Design review of the part shown in the three views and the two pictorial views. Dimensions are in mm from the part's minimum x, y and z. Round coordinates to 2 decimals unless told otherwise and drop trailing zeros. Order: outer loops, then holes, each group sorted by start corner. A loop starts at its lowest first (then second) coordinate and runs counter-clockwise, first axis right, second up.
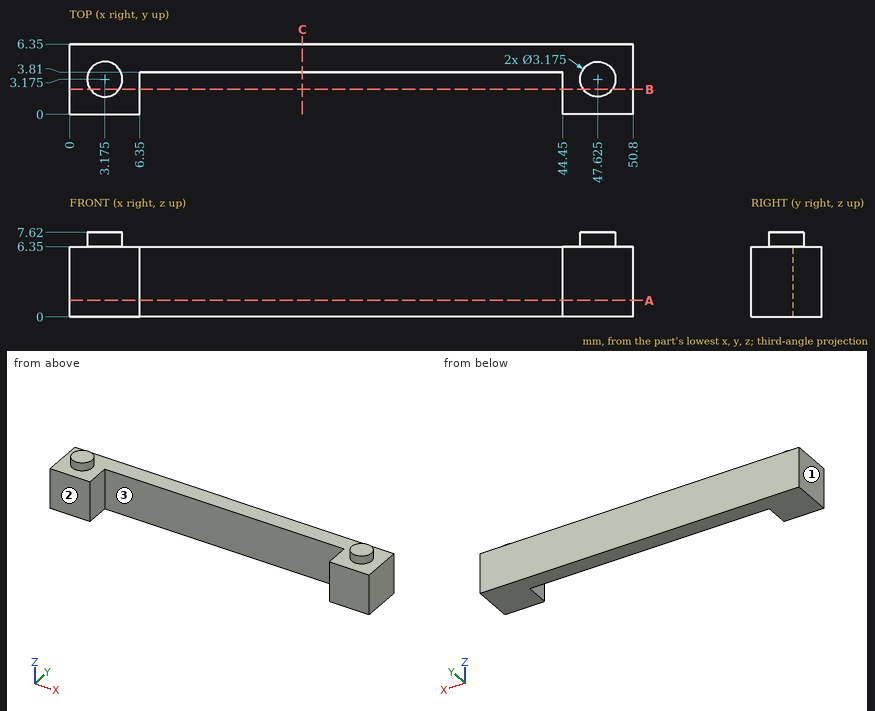
(1) Draft analysis for pull direction X (two halves, no side actions). For the marked faces 1, 2 and 3, state which applies: pulls with the +X half, pulls with the -X half, needs draft (parallel to the pull), parting line crosses it, or undercut.
(2) Clearance check with flat-ended pins moving along their axes: P1, Ø3, axis at x = 29, z = 1, coming from the -Y side; P2, Ø3, axis at x = 27, y = 5.5, coming from the +Z side. State where each tip first meets the part, or that it passes through.
(3) Add section A-A on z = 1.5. Give the boundary of the cut face in (x, y).
(4) Wall thickness on L1, parallel to X at y = 0.75, z = 3.5; L2, parallel to Z at x = 38, y = 5.5; L3, parallel to Y at x = 28.5, z = 5.75: over which ranges is each line inside the solid? List them lowest first.
(5) Add section C-C on x = 21. Give the boundary of the cut face in (y, z).
(6) Add section B-B on y = 2.25. Give the boundary of the cut face in (x, z).
Here are the results:
1. face 1: pulls with the -X half
1. face 2: needs draft
1. face 3: undercut
2. P1: stops at y = 3.81
2. P2: stops at z = 6.35
3. outline: (0, 0) - (6.35, 0) - (6.35, 3.81) - (44.45, 3.81) - (44.45, 0) - (50.8, 0) - (50.8, 6.35) - (0, 6.35) - close
4. L1: x = 0 to 6.35, 44.45 to 50.8
4. L2: z = 0 to 6.35
4. L3: y = 3.81 to 6.35
5. outline: (3.81, 0) - (6.35, 0) - (6.35, 6.35) - (3.81, 6.35) - close
6. outline: (0, 0) - (6.35, 0) - (6.35, 6.35) - (4.47, 6.35) - (4.47, 7.62) - (1.88, 7.62) - (1.88, 6.35) - (0, 6.35) - close; (44.45, 0) - (50.8, 0) - (50.8, 6.35) - (48.92, 6.35) - (48.92, 7.62) - (46.33, 7.62) - (46.33, 6.35) - (44.45, 6.35) - close
